Work out the finished part from the listing and answer in its coordinate system (mm). A direction names the side the tool comes from. Coordinates: 2 decimals unless noted, no trailing zeros. Write each loop counter-clockwise with the first axis right and the second up, starting at its lowest first coordinate (ties: lowest second). Pieces come first, ordered by that corner, then holes. Notation, with made-up numbers: (-6.5, 22.25) - (44.5, 22.25) arc R23 ccw to (44.5, 40.25) - close; hole circle Ø8 at (-39.75, -37.5). An arc over 180 degrees is marked (long way). Use a Markdown table: item, result. Add a question column.
(1) The part is cut by section D-D, the plane z = 2. State how many separate pieces and enclosed holes the cut face has, then the cut area to 3 significant figures.
(2) Find the intervals of material crossed by line 1 (Y direction, x = 0, z = 11); line 2 (Z direction, x = 9, y = 14); line 3 (X direction, y = 3.5, z = 19.5), in increasing order. Write a range as from..to.
(3) The part is cut by section A-A, the plane x = 0. Give the vertices of the cut face in (y, z) (3 decimals), then the cut area to 3 significant figures.
(4) For a pull along Y with two mould halves and no side action, classify faces 4 (the face through (-28.547, -1.256, 2.254)), 5 (the face through (12, -6, 4.572)), 6 (the face through (-23.118, -11.12, 2.254)) as released by +Y, released by -Y, zero draft, split by the parting line, or undercut.
(5) Given pin 1 Ø5 at (x, y) = (8.5, -20.5) entering from +Z; pin 2 Ø3 at (y, z) = (-10.5, 22) entering from +X; pin 3 Ø4 at (y, z) = (7, 9) entering from +X, each flat-ended and moving along its own axis, determine where each tip first touches the part or whether it passes through.
(6) The part is cut by section C-C, the plane y = 0. Give the vertices of the cut face in (x, z) (3 decimals), then the cut area to 3 significant figures.
(7) The part is cut by section B-B, the plane z = 18.5. Give the vertices of the cut face in (x, y).
(8) A tool of negligible diameter and unlimited length cuts with its end or side. For faces 1 (the face through (-0.2, -5.2, 25.4)), 2 (the face through (-2, -12, 15)), 3 (the face through (0, 6.091, 13)), from which of +Z, -Z, +X, -X, +Y, -Y can it reach the whole face along a straight path? Write none if from no direction.
Autodesk Inventor part; units mm, degrees
ref_plane "YZ Plane" through (0, 0, 0) normal (1, 0, 0) x (0, 1, 0)
ref_plane "XZ Plane" through (0, 0, 0) normal (0, 1, 0) x (-1, 0, 0)
ref_plane "XY Plane" through (0, 0, 0) normal (0, 0, 1) x (1, 0, 0)
sketch "Sketch1" plane through (0, 0, 0) normal (0, 0, 1) x (1, 0, 0)
  circle A0 centre (0, 0) radius 28.575
  dimension "d0" = 57.15
extrude "Extrusion1" add sketch "Sketch1" along normal blind 4.572
sketch "Sketch2" plane through (0, 0, 4.572) normal (0, 0, 1) x (1, 0, 0)
  circle A0 centre (0, 0) radius 28.575
  circle A1 centre (0, 0) radius 12.1666
  dimension "d3" = 24.3332
extrude "Extrusion2" add sketch "Sketch2" along normal blind 20.828 contours A1
sketch "Sketch3" plane through (0, 0, 25.4) normal (0, 0, 1) x (1, 0, 0)
  circle A0 centre (0, 0) radius 12.1666
  circle A1 centre (0, 0) radius 5
  line L0 (-1.25, 6.0912) -> (1.25, 6.0912)
  line L1 (1.25, 6.0912) -> (1.25, 3.5912)
  line L2 (1.25, 3.5912) -> (-1.25, 3.5912)
  line L3 (-1.25, 3.5912) -> (-1.25, 6.0912)
  point P0 (0, 6.0912)
  point P1 (-1.25, 4.8412)
  dimension "d6" = 10
  dimension "d7" = 2.5
  dimension "d8" = 2.5
extrude "Extrusion3" cut sketch "Sketch3" against normal through all contours A1 L3 L2 L1 | L1 L2 L3 A1 | A1 L3 L0 L1
sketch "Sketch4" plane through (0, 0, 0) normal (0, 0, -1) x (-1, 0, 0)
  arc A0 (-1.25, 4.8412) -> (1.25, 4.8412) centre (0, 0) ccw
  circle A1 centre (0, 23.8125) radius 2.6162
  arc A2 (-1.25, 4.8412) -> (1.25, 4.8412) centre (0, 0) ccw
  line L0 (-1.25, 4.8412) -> (-1.25, 6.0912)
  line L1 (-1.25, 6.0912) -> (1.25, 6.0912)
  line L2 (1.25, 6.0912) -> (1.25, 4.8412)
  circle A3 centre (0, 0) radius 28.575
  dimension "d11" = 5.2324
  dimension "d12" = 23.8125
extrude "Extrusion4" cut sketch "Sketch4" against normal through all contours A1
pattern_circular "Circular Pattern1" count 6 over 360 about axis through (0, 0, 0) along (0, 0, 1) of "Extrusion4"
properties part number "Hub 8mm key"
Model answer:
| question | item | result |
|---|---|---|
| 1 | separate pieces | 1 |
| 1 | enclosed holes | 7 |
| 1 | area | 2,350 mm^2 |
| 2 | line 1 | -12.17..-5, 6.09..12.17 |
| 2 | line 2 | 0..4.57 |
| 2 | line 3 | -11.65..-3.57, 3.57..11.65 |
| 3 | outline | (-28.575, 0) - (-26.429, 0) - (-26.429, 4.572) - (-28.575, 4.572) - close; (-21.196, 0) - (-5, 0) - (-5, 25.4) - (-12.167, 25.4) - (-12.167, 4.572) - (-21.196, 4.572) - close; (6.091, 0) - (21.196, 0) - (21.196, 4.572) - (12.167, 4.572) - (12.167, 25.4) - (6.091, 25.4) - close; (26.429, 0) - (28.575, 0) - (28.575, 4.572) - (26.429, 4.572) - close |
| 3 | area | 439 mm^2 |
| 4 | face 4 | split by the parting line |
| 4 | face 5 | zero draft |
| 4 | face 6 | undercut |
| 5 | pin 1 | z = 4.57 |
| 5 | pin 2 | x = 8.19 |
| 5 | pin 3 | x = 11.09 |
| 6 | outline | (-28.575, 0) - (-5, 0) - (-5, 25.4) - (-12.167, 25.4) - (-12.167, 4.572) - (-28.575, 4.572) - close; (5, 0) - (28.575, 0) - (28.575, 4.572) - (12.167, 4.572) - (12.167, 25.4) - (5, 25.4) - close |
| 6 | area | 514 mm^2 |
| 7 | outline | circle Ø24.33 at (0, 0); hole (-1.25, 4.84) arc R5 ccw (long way) to (1.25, 4.84) - (1.25, 6.09) - (-1.25, 6.09) - close |
| 8 | face 1 | +Z, +X, -X, +Y, -Y |
| 8 | face 2 | +Z |
| 8 | face 3 | +Z, -Z |
